Check sheet for the modelled part. Datum: model origin and axes. Units: mm. A direction names the side the tool comes from. Give positions to 0.01 mm unless a question says otherwise; leave off trailing zeros. Loops run counter-clockwise (first coordinate to the right, second up) from the corner with the lowest first, then second, coordinate; pieces in that order, holes last. Notation, with made-up numbers: (-3.75, 78.25) - (39.25, 78.25) arc R12 cw to (39.25, 98.25) - close; hole circle Ø1 at (64.5, -37.75). An arc over 180 degrees is marked (long way). Use one line per item in the form item = value.
from build123d import *

# Parameters (mm, degrees)
SKETCH1_R           = 60
BOSS_EXTRUDE1_DEPTH = 17
SKETCH2_R           = 52
SKETCH2_R_2         = 22
CUT_EXTRUDE1_DEPTH  = 4
FILLET1_R           = 5
CHAMFER1_SIZE       = 2
SKETCH3_R           = 15
CUT_EXTRUDE2_DEPTH  = 87.539008545


with BuildPart() as part:
    # Sketch1 → Boss-Extrude1 (new body)
    with BuildSketch(Plane(origin=(0, 0, 0), x_dir=(1, 0, 0), z_dir=(0, 1, 0))):
        with Locations(Location((0, 0, 0), (0, 0, 270))):
            Circle(SKETCH1_R)
    extrude(amount=BOSS_EXTRUDE1_DEPTH)

    # Sketch2 → Cut-Extrude1 (cut)
    with BuildSketch(Plane(origin=(0, 17, 0), x_dir=(1, 0, 0), z_dir=(0, 1, 0))):
        with Locations(Location((0, 0, 0), (0, 0, 270))):
            Circle(SKETCH2_R)
        with Locations(Location((0, 0, 0), (0, 0, 270))):
            Circle(SKETCH2_R_2, mode=Mode.SUBTRACT)
    cut_extrude1 = extrude(amount=-CUT_EXTRUDE1_DEPTH, mode=Mode.SUBTRACT)

    # Mirror1: Cut-Extrude1 across plane
    add(cut_extrude1.mirror(Plane.ZX.offset(8.5)), mode=Mode.SUBTRACT)

    # Fillet1
    # the kernel refuses this fillet: 5 mm, written as the material it adds along each edge
    with BuildSketch(Plane(origin=(0, 4, 0), x_dir=(0, 0, 1), z_dir=(-1, 0, 0))) as fillet1_piece_1:
        with BuildLine():
            CenterArc((47.101020514, -5), FILLET1_R, 11.536959033, 78.463040967)
            Line((47.101020514, 0), (47.101020514, 0.1))
            Line((47.101020514, 0.1), (52, 0.1))
            Line((52, 0.1), (52.1, 0))
            ThreePointArc((52.1, 0), (52.1, -2), (52.09797959, -3.98))
            Line((52.09797959, -3.98), (52, -4))
        make_face()
    revolve(axis=Axis((0, 4, 0), (0, 1, 0)))
    with BuildSketch(Plane(origin=(0, 4, 0), x_dir=(0, 0, 1), z_dir=(-1, 0, 0))) as fillet1_piece_2:
        with BuildLine():
            CenterArc((26.898979486, -5), FILLET1_R, 90, 78.463040967)
            Line((22, -4), (21.90202041, -3.98))
            ThreePointArc((21.90202041, -3.98), (21.9, -2), (21.9, 0))
            Line((21.9, 0), (22, 0.1))
            Line((22, 0.1), (26.898979486, 0.1))
            Line((26.898979486, 0.1), (26.898979486, 0))
        make_face()
    revolve(axis=Axis((0, 4, 0), (0, 1, 0)))
    with BuildSketch(Plane(origin=(0, 13, 0), x_dir=(0, 0, 1), z_dir=(-1, 0, 0))) as fillet1_piece_3:
        with BuildLine():
            CenterArc((47.101020514, 5), FILLET1_R, 270, 78.463040967)
            Line((47.101020514, 0), (47.101020514, -0.1))
            Line((47.101020514, -0.1), (52, -0.1))
            Line((52, -0.1), (52.1, 0))
            ThreePointArc((52.1, 0), (52.1, 2), (52.09797959, 3.98))
            Line((52.09797959, 3.98), (52, 4))
        make_face()
    revolve(axis=Axis((0, 13, 0), (0, 1, 0)))
    with BuildSketch(Plane(origin=(0, 13, 0), x_dir=(0, 0, 1), z_dir=(-1, 0, 0))) as fillet1_piece_4:
        with BuildLine():
            CenterArc((26.898979486, 5), FILLET1_R, 191.536959033, 78.463040967)
            Line((22, 4), (21.90202041, 3.98))
            ThreePointArc((21.90202041, 3.98), (21.9, 2), (21.9, 0))
            Line((21.9, 0), (22, -0.1))
            Line((22, -0.1), (26.898979486, -0.1))
            Line((26.898979486, -0.1), (26.898979486, 0))
        make_face()
    revolve(axis=Axis((0, 13, 0), (0, 1, 0)))

    # Chamfer1
    chamfer1_edges = [part.edges().sort_by_distance(p)[0] for p in [
        (0, 0, -60),
        (0, 17, -60),
    ]]
    chamfer(chamfer1_edges, length=CHAMFER1_SIZE)

    # Sketch3 → Cut-Extrude2 (cut, through all)
    with BuildSketch(Plane.XZ):
        with Locations(Location((0, 0, 0), (0, 0, 270))):
            Circle(SKETCH3_R)
    extrude(amount=-CUT_EXTRUDE2_DEPTH, mode=Mode.SUBTRACT)


solid = part.part
Item 1: Access from +Z, -Z, +X, -X, +Y, -Y to the whole of each face (thin tool, end or side, straight path). Record for faces 1 (the face through (-20, 4, 20)), 2 (the face through (-20, 13, 20)), 3 (the face through (48, 0, -22)).
Answer block:
face_1 = -Y
face_2 = +Y
face_3 = +Z, -Z, +X, -X, -Y
Item 2: Section check B-B on z = 0. Record the boundary of the cut face in (x, y).
Answer block:
outline = (-60, 2) - (-58, 0) - (-52, 0) arc R5 cw to (-47.1, 4) - (-26.9, 4) arc R5 cw to (-22, 0) - (-15, 0) - (-15, 17) - (-22, 17) arc R5 cw to (-26.9, 13) - (-47.1, 13) arc R5 cw to (-52, 17) - (-58, 17) - (-60, 15) - close; (15, 0) - (22, 0) arc R5 cw to (26.9, 4) - (47.1, 4) arc R5 cw to (52, 0) - (58, 0) - (60, 2) - (60, 15) - (58, 17) - (52, 17) arc R5 cw to (47.1, 13) - (26.9, 13) arc R5 cw to (22, 17) - (15, 17) - close
Item 3: Section check C-C on y = 5.5. Record the boundary of the cut face in (x, z).
Answer block:
outline = circle Ø120 at (0, 0); hole circle Ø30 at (0, 0)
Item 4: Mould release check, pull along X, two halves, no side actions. Record for faces 4 (the face through (57.63, 16.875, -7.567)), 5 (the face through (48, 17, -22)), 6 (the face through (0.66, 8.381, 14.985)): released by +X, released by -X, zero draft, split by the parting line, or undercut.
Answer block:
face_4 = split by the parting line
face_5 = zero draft
face_6 = undercut
Item 5: Gauge pin test, flat ends, axial feed: P1, Ø8, axis at x = -39.5, y = 3.5, coming from the -Z side; P2, Ø1, axis at x = -5.5, y = 15, coming from the -Z side; P3, Ø3, axis at x = 13, y = 7.5, coming from the +Z side. Record the tip position at first contact, or that the pin passes through.
Answer block:
P1 = -48.37
P2 = -59.79
P3 = 58.89
Item 6: Thickness scan on L1, parallel to Z at x = 1, y = 7; L2, parallel to X at y = 11.5, z = 0; L3, parallel to Z at x = 17.5, y = 15.5. Record the ranges inside material, lowest first.
Answer block:
L1 = -59.99 to -14.97, 14.97 to 59.99
L2 = -60 to -15, 15 to 60
L3 = -56.87 to -48.36, -14.25 to 14.25, 48.36 to 56.87
Item 7: Section check A-A on x = 0. Record the boundary of the cut face in (y, z), then the cut area to 3 significant figures.
Answer block:
outline = (0, -58) - (2, -60) - (15, -60) - (17, -58) - (17, -52) arc R5 cw to (13, -47.1) - (13, -26.9) arc R5 cw to (17, -22) - (17, -15) - (0, -15) - (0, -22) arc R5 cw to (4, -26.9) - (4, -47.1) arc R5 cw to (0, -52) - close; (0, 15) - (17, 15) - (17, 22) arc R5 cw to (13, 26.9) - (13, 47.1) arc R5 cw to (17, 52) - (17, 58) - (15, 60) - (2, 60) - (0, 58) - (0, 52) arc R5 cw to (4, 47.1) - (4, 26.9) arc R5 cw to (0, 22) - close
area = 1,080 mm2
